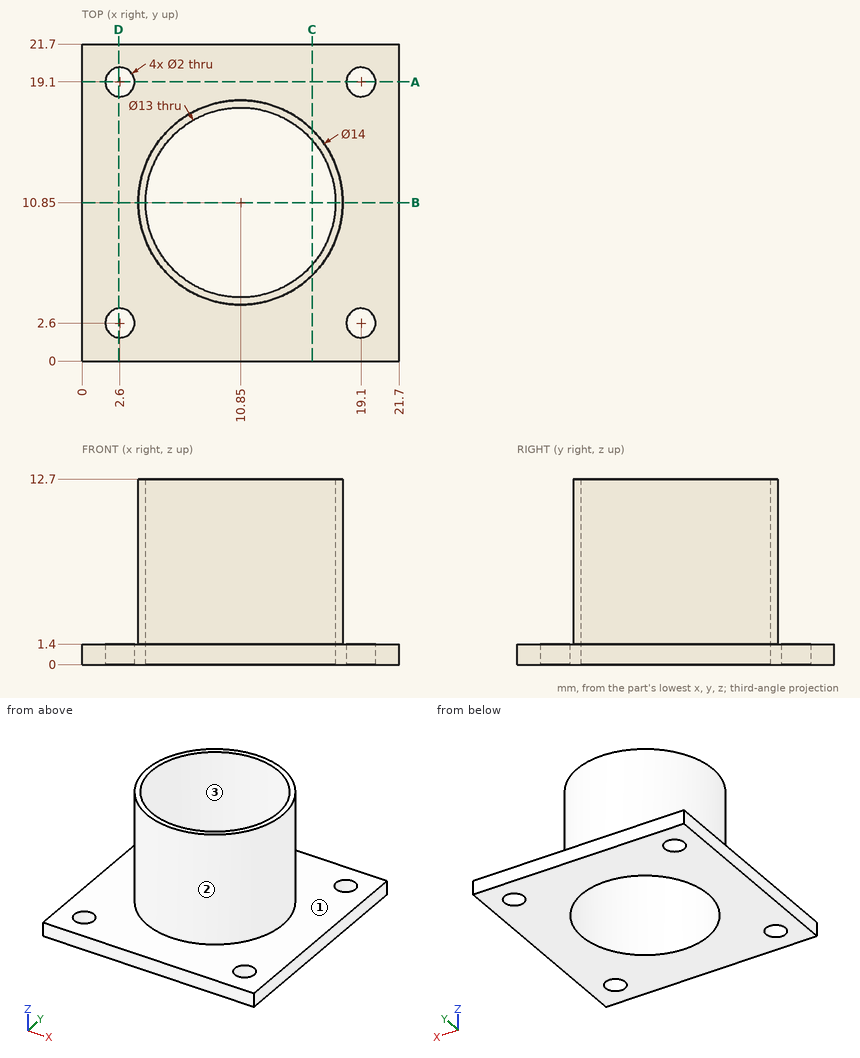
Input: dimensioned drawing with shaded views. Units: mm. Origin: part minimum x, y, z. Round coordinates to 2 decimals unless told otherwise and drop trailing zeros. Loops run counter-clockwise (first coordinate to the right, second up) from the corner with the lowest first, then second, coordinate; pieces in that order, holes last. Notation, with made-up numbers: (10.5, 1.5) -> (60.5, 1.5) arc R23 ccw to (60.5, 20.5) -> close; hole circle Ø11 at (72, -30.75). An arc over 180 degrees is marked (long way). Answer as a JSON object with one key per item and string values. Group by question number.
Q1. Ray query, line 1 (Y direction, x = 2.6, z = 0.95); line 2 (Y direction, x = 10.85, z = 3.5); line 3 (Z direction, x = 8.5, y = 18.5). Return the intervals inside material, ascending. Write a range as from..to.
Q2. Section query B-B (y = 10.85). Output: boundary loops of the cut face in (x, z), plus the area to 3 significant figures.
Q3. Section query C-C (x = 15.75). Output: boundary loops of the cut face in (y, z).
Q4. Contact query for flat-ended pins moving along their axis: P1, Ø4, axis at y = 14.5, z = 7, coming from the -X side; P2, Ø3, axis at x = 15, z = 4.5, coming from the +Y side; P3, Ø1.5, axis at x = 17, z = 11, coming from the +Y side; P4, Ø1.5, axis at x = 10, y = 15.5, coming from the -Z side. Output: stop coordinate, or through.
Q5. Mould query, pull axis X, two halves, no side actions, for the marked faces 1, 2 and 3. Classes: pulls with the +X half, pulls with the -X half, needs draft (parallel to the pull), parting line crosses it, or undercut.
Q6. Section query D-D (x = 2.5). Output: boundary loops of the cut face in (y, z), plus the area to 3 significant figures.
Q7. Section query A-A (y = 19.1). Output: boundary loops of the cut face in (x, z).
Completed:
{
 "1": {"line 1": "0..1.6, 3.6..18.1, 20.1..21.7", "line 2": "3.85..4.35, 17.35..17.85", "line 3": "0..1.4"},
 "2": {"outline": "(0, 0) -> (4.35, 0) -> (4.35, 12.7) -> (3.85, 12.7) -> (3.85, 1.4) -> (0, 1.4) -> close; (17.35, 0) -> (21.7, 0) -> (21.7, 1.4) -> (17.85, 1.4) -> (17.85, 12.7) -> (17.35, 12.7) -> close", "area": "23.5 mm²"},
 "3": {"outline": "(0, 0) -> (6.58, 0) -> (6.58, 12.7) -> (5.85, 12.7) -> (5.85, 1.4) -> (0, 1.4) -> close; (15.12, 0) -> (21.7, 0) -> (21.7, 1.4) -> (15.85, 1.4) -> (15.85, 12.7) -> (15.12, 12.7) -> close"},
 "4": {"P1": "x = 4.05", "P2": "y = 17.33", "P3": "y = 15.3", "P4": "through"},
 "5": {"face 1": "needs draft", "face 2": "parting line crosses it", "face 3": "undercut"},
 "6": {"outline": "(0, 0) -> (1.61, 0) -> (1.61, 1.4) -> (0, 1.4) -> close; (3.59, 0) -> (18.11, 0) -> (18.11, 1.4) -> (3.59, 1.4) -> close; (20.09, 0) -> (21.7, 0) -> (21.7, 1.4) -> (20.09, 1.4) -> close", "area": "24.8 mm²"},
 "7": {"outline": "(0, 0) -> (1.6, 0) -> (1.6, 1.4) -> (0, 1.4) -> close; (3.6, 0) -> (18.1, 0) -> (18.1, 1.4) -> (3.6, 1.4) -> close; (20.1, 0) -> (21.7, 0) -> (21.7, 1.4) -> (20.1, 1.4) -> close"}
}
